Read the model definition and answer for the solid it produces. Units are mm, in the model's axes. A direction names the side the tool comes from. Coordinates: 2 decimals unless noted, no trailing zeros. Order: outer loops, then holes, each group sorted by start corner. A loop starts at its lowest first (then second) coordinate and runs counter-clockwise, first axis right, second up.
from build123d import *

# Parameters (mm, degrees)
IZIM1_R                           = 3
Y_KSEKLIK_EKSTR_ZYON1_DEPTH       = 6
IZIM2_R                           = 5
IZIM2_R_2                         = 3
Y_KSEKLIK_EKSTR_ZYON2_DEPTH       = 6
Y_KSEKLIK_EKSTR_ZYON3_DEPTH       = 1.5
KES_EKSTR_ZYON1_REACH             = 31.585
IZIM5_R                           = 3.5
KES_EKSTR_ZYON1_DIRECTION_2_REACH = 31.585
IZIM6_R                           = 2.838174874
KES_EKSTR_ZYON2_DEPTH             = 44
PAH1_SIZE                         = 1


with BuildPart() as part:
    # Çizim1 → Yükseklik-Ekstrüzyon1 (new body)
    with BuildSketch(Plane(origin=(0, 0, 0), x_dir=(1, 0, 0), z_dir=(0, 1, 0))):
        with BuildLine():
            Line((-16.5, 15), (16.5, 15))
            ThreePointArc((16.5, 15), (20.742640687, 13.242640687), (22.5, 9))
            Line((22.5, 9), (22.5, -9))
            ThreePointArc((22.5, -9), (20.742640687, -13.242640687), (16.5, -15))
            Line((16.5, -15), (-16.5, -15))
            ThreePointArc((-16.5, -15), (-20.742640687, -13.242640687), (-22.5, -9))
            Line((-22.5, -9), (-22.5, 9))
            ThreePointArc((-22.5, 9), (-20.742640687, 13.242640687), (-16.5, 15))
        make_face()
        with Locations(Location((0, 0, 0), (0, 0, 270))):
            Circle(IZIM1_R, mode=Mode.SUBTRACT)
    extrude(amount=Y_KSEKLIK_EKSTR_ZYON1_DEPTH)

    # Çizim2 → Yükseklik-Ekstrüzyon2 (add)
    with BuildSketch(Plane(origin=(0, 6, 0), x_dir=(1, 0, 0), z_dir=(0, 1, 0))):
        with Locations(Location((0, 0, 0), (0, 0, 270))):
            Circle(IZIM2_R)
        with Locations(Location((0, 0, 0), (0, 0, 270))):
            Circle(IZIM2_R_2, mode=Mode.SUBTRACT)
    extrude(amount=Y_KSEKLIK_EKSTR_ZYON2_DEPTH)

    # Çizim4 → Yükseklik-Ekstrüzyon3 (add, symmetric)
    with BuildSketch(Plane.XY):
        Polygon((-5.65775064, 12), (-3.798545346, 12), (-3.798545346, 6), (-9.121852255, 6), align=None)
        Polygon((3.798545346, 12), (3.798545346, 6), (9.121852255, 6), (5.65775064, 12), align=None)
    extrude(amount=Y_KSEKLIK_EKSTR_ZYON3_DEPTH, both=True)

    # Kes-Ekstrüzyon1: up to this face of the body (flat: up to its plane)
    kes_ekstr_zyon1_end = Plane(part.part.faces().sort_by_distance((-22.5, 3, 0))[0])
    # Çizim5 → Kes-Ekstrüzyon1 (cut, up to the picked face)
    with BuildSketch(Plane(origin=(0, 0, 0), x_dir=(0, 0, -1), z_dir=(1, 0, 0)), mode=Mode.PRIVATE) as kes_ekstr_zyon1_sk1:
        with Locations((-10, 0)):
            Circle(IZIM5_R)
    kes_ekstr_zyon1_tool1 = split(extrude(kes_ekstr_zyon1_sk1.sketch, amount=-KES_EKSTR_ZYON1_REACH, mode=Mode.PRIVATE), bisect_by=kes_ekstr_zyon1_end, keep=Keep.BOTH, mode=Mode.PRIVATE)
    add(kes_ekstr_zyon1_tool1.solids().sort_by(Axis((0, 0, 10), (-1, 0, 0)))[0], mode=Mode.SUBTRACT)

    # Kes-Ekstrüzyon1 direction 2: up to this face of the body (flat: up to its plane)
    kes_ekstr_zyon1_direction_2_end = Plane(part.part.faces().sort_by_distance((22.5, 3, 0))[0])
    # Çizim5 → Kes-Ekstrüzyon1 direction 2 (cut, up to the picked face)
    with BuildSketch(Plane(origin=(0, 0, 0), x_dir=(0, 0, -1), z_dir=(1, 0, 0)), mode=Mode.PRIVATE) as kes_ekstr_zyon1_direction_2_sk1:
        with Locations((-10, 0)):
            Circle(IZIM5_R)
    kes_ekstr_zyon1_direction_2_tool1 = split(extrude(kes_ekstr_zyon1_direction_2_sk1.sketch, amount=KES_EKSTR_ZYON1_DIRECTION_2_REACH, mode=Mode.PRIVATE), bisect_by=kes_ekstr_zyon1_direction_2_end, keep=Keep.BOTH, mode=Mode.PRIVATE)
    add(kes_ekstr_zyon1_direction_2_tool1.solids().sort_by(Axis((0, 0, 10), (1, 0, 0)))[0], mode=Mode.SUBTRACT)

    # Çizim6 → Kes-Ekstrüzyon2 (cut)
    with BuildSketch(Plane.XZ):
        with Locations(Location((-12.5, -5, 0), (0, 0, 270))):
            Circle(IZIM6_R)
        with Locations(Location((12.5, -5, 0), (0, 0, 270))):
            Circle(IZIM6_R)
    extrude(amount=-KES_EKSTR_ZYON2_DEPTH, mode=Mode.SUBTRACT)

    # Pah1
    pah1_edges = [part.edges().sort_by_distance(p)[0] for p in [
        (-12.5, 6, -2.161825126),
        (-12.5, 0, -2.161825126),
        (12.5, 6, -2.161825126),
        (12.5, 0, -2.161825126),
    ]]
    chamfer(pah1_edges, length=PAH1_SIZE)


solid = part.part
Q1. Which of the six approach directions +Z, -Z, +X, -X, +Y, -Y give full straight-line access (tool end or side, diameter ignored) to faces 1 (the flat face through (-6, 8, -1.5)), 2 (the cylindrical face through (0, 9, -5)), 3 (the cylindrical face through (0, 9, 5))?
Q2. Determine the mould class of faces 4 (the cylindrical face through (10.77, 2.97, -2.75)), 5 (the flat face through (5, 6, 3)), 6 (the cylindrical face through (20.696, 2.958, -13.289)) for opening direction Z: +Z half, -Z half, draft (parallel to the pull), parting line (faces both ways), or undercut.
Q3. The part is cut by section A-A, the plane z = 0. Determine the outline of the cut face in (x, y), then the cut area to 3 significant figures.
Q4. The part is cut by section D-D, the plane x = -19.5. Determine the outline of the cut face in (y, z), then the cut area to 3 significant figures.
Q5. The part is cut by section C-C, the plane y = 7.5. Determine the outline of the cut face in (x, z), then the cut area to 3 significant figures.
Q6. Each of these flat-tipped pins is pushed along its axis until it touches: P1, Ø5, axis at x = 7, y = 8, coming from the -Z side; P2, Ø1.3, axis at x = -7, y = 8, coming from the -Z side; P3, Ø1.3, axis at x = -7, y = 8, coming from the +Z side; P4, Ø6.5, axis at x = 12.5, z = -5, coming from the +Y side. Where does it stop, or does it pass through?
Q7. The part is cut by section B-B, the plane x = 12.5. Determine the outline of the cut face in (y, z).
Q8. Straight lines are drawn through the part: L1, parallel to X at y = 2.2, z = -5; L2, parallel to Y at x = 7, z = -8; L3, parallel to Y at x = 16, z = 10. For each, find the intervals that lie inside material, in ascending order.
Computed values:
1. face 1: -Z, -X, +Y
1. face 2: -Z, +Y
1. face 3: +Z, +Y
2. face 4: undercut
2. face 5: draft
2. face 6: -Z half
3. outline: (-22.5, 0) - (-3, 0) - (-3, 12) - (-5.66, 12) - (-9.12, 6) - (-22.5, 6) - close; (3, 0) - (22.5, 0) - (22.5, 6) - (9.12, 6) - (5.66, 12) - (3, 12) - close
3. area: 287 mm2
4. outline: (0, -14.2) - (6, -14.2) - (6, 14.2) - (0, 14.2) - (0, 13.5) arc R3.5 cw to (0, 6.5) - close
4. area: 151 mm2
5. outline: (-8.26, -1.5) - (-4.77, -1.5) arc R5 ccw to (4.77, -1.5) - (8.26, -1.5) - (8.26, 1.5) - (4.77, 1.5) arc R5 ccw to (-4.77, 1.5) - (-8.26, 1.5) - close; hole circle Ø6 at (0, 0)
5. area: 70.3 mm2
6. P1: stops at z = -15
6. P2: stops at z = -1.5
6. P3: stops at z = 1.5
6. P4: stops at y = 5.41
7. outline: (0, -15) - (6, -15) - (6, -8.84) - (5, -7.84) - (1, -7.84) - (0, -8.84) - close; (0, -1.16) - (1, -2.16) - (5, -2.16) - (6, -1.16) - (6, 15) - (0, 15) - (0, 13.5) arc R3.5 cw to (0, 6.5) - close
8. L1: x = -22.5 to -15.34, -9.66 to 9.66, 15.34 to 22.5
8. L2: y = 0 to 6
8. L3: y = 3.5 to 6
